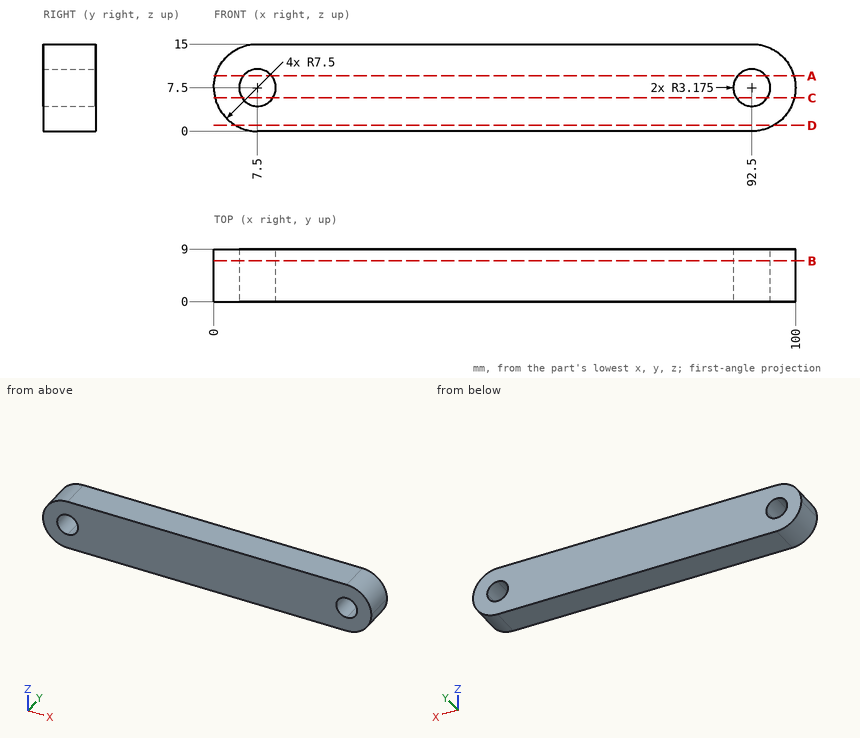
Job drawing, mm, ordinate dimensions from the low corner. One solid piece. Coordinates: 2 decimals unless noted, no trailing zeros. Order: outer loops, then holes, each group sorted by start corner. A loop starts at its lowest first (then second) coordinate and runs counter-clockwise, first axis right, second up. Notation, with made-up numbers: (73, 39.25) -> (127, 39.25) arc R16 cw to (127, 46.25) -> close; hole circle Ø1 at (53, 6.5). An arc over 180 degrees is marked (long way). Return JSON: item names as keys, results as strings. Group by question number.
Item 1: Saw through at C-C on z = 5.75. Write the cut outline in (x, y), then the cut area to 3 significant figures.
Item 2: Wall check: line 1 along X through (y, z) = (0.75, 8.75) (1 decimal); line 2 along X through (y, z) = (6.5, 2.75); line 3 along X through (y, z) = (3.25, 1.25). Give the ranges that are in metal, low to high. Write a range as [from, to].
Item 3: Saw through at B-B on y = 7. State how many separate pieces and enclosed holes the cut face has, then the cut area to 3 significant figures.
Item 4: Saw through at A-A on z = 9.5. Write the cut outline in (x, y), then the cut area to 3 significant figures.
Item 5: Saw through at D-D on z = 1. Write the cut outline in (x, y), then the cut area to 3 significant figures.
Values found:
{
 "1": {"outline": "(0.21, 0) -> (4.85, 0) -> (4.85, 9) -> (0.21, 9) -> close; (10.15, 0) -> (89.85, 0) -> (89.85, 9) -> (10.15, 9) -> close; (95.15, 0) -> (99.79, 0) -> (99.79, 9) -> (95.15, 9) -> close", "area": "801 mm2"},
 "2": {"line 1": "x = [0.1, 4.6], [10.4, 89.6], [95.4, 99.9]", "line 2": "x = [1.7, 98.3]", "line 3": "x = [3.35, 96.65]"},
 "3": {"separate pieces": "1", "enclosed holes": "2", "area": "1,390 mm2"},
 "4": {"outline": "(0.27, 0) -> (5.03, 0) -> (5.03, 9) -> (0.27, 9) -> close; (9.97, 0) -> (90.03, 0) -> (90.03, 9) -> (9.97, 9) -> close; (94.97, 0) -> (99.73, 0) -> (99.73, 9) -> (94.97, 9) -> close", "area": "806 mm2"},
 "5": {"outline": "(3.76, 0) -> (96.24, 0) -> (96.24, 9) -> (3.76, 9) -> close", "area": "832 mm2"}
}
